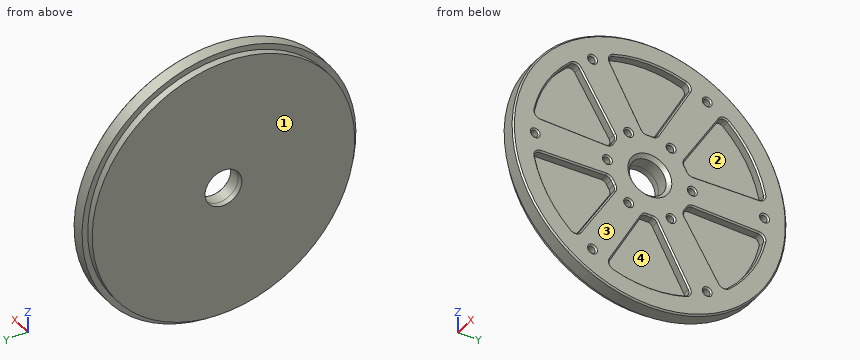
```python
from build123d import *

# Parameters (mm, degrees)
SKETCH1_R           = 48.35
BOSS_EXTRUDE1_DEPTH = 2.725
SKETCH3_R           = 1.25
CUT_EXTRUDE1_DEPTH  = 3
CIRPATTERN1_COUNT   = 6
SKETCH4_R           = 1.25
CUT_EXTRUDE2_DEPTH  = 3
CIRPATTERN2_COUNT   = 6
SKETCH5_R           = 6.5
CUT_EXTRUDE3_DEPTH  = 5.45
CHAMFER1_SIZE       = 0.5
CHAMFER2_SIZE       = 1.25
CHAMFER3_SIZE       = 0.5
SKETCH6_R           = 46.35
SKETCH6_R_2         = 6.5
BOSS_EXTRUDE2_DEPTH = 2
CUT_EXTRUDE4_START  = -0.5
SKETCH7_R           = 48.35
SKETCH7_R_2         = 46.35
CUT_EXTRUDE4_DEPTH  = 0.5
CUT_EXTRUDE6_DEPTH  = 3
CIRPATTERN3_COUNT   = 6
CHAMFER4_SIZE       = 0.5


with BuildPart() as part:
    # Sketch1 → Boss-Extrude1 (new, symmetric)
    with BuildSketch(Plane(origin=(0, 0, 0), x_dir=(0, 0, -1), z_dir=(1, 0, 0))):
        Circle(SKETCH1_R)
    extrude(amount=BOSS_EXTRUDE1_DEPTH, both=True)

    # Sketch3 → Cut-Extrude1 (cut)
    with BuildSketch(Plane(origin=(2.725, 0, 0), x_dir=(0, 0, -1), z_dir=(1, 0, 0))):
        with Locations((0, 40.5)):
            Circle(SKETCH3_R)
    cut_extrude1 = extrude(amount=-CUT_EXTRUDE1_DEPTH, mode=Mode.SUBTRACT)

    # CirPattern1: Cut-Extrude1 ×6 about axis
    cirpattern1_axis = Axis((0, 0, 0), (1, 0, 0))
    for i in range(1, CIRPATTERN1_COUNT):
        add(cut_extrude1.rotate(cirpattern1_axis, i * 360 / CIRPATTERN1_COUNT), mode=Mode.SUBTRACT)

    # Sketch4 → Cut-Extrude2 (cut)
    with BuildSketch(Plane(origin=(2.725, 0, 0), x_dir=(0, 0, -1), z_dir=(1, 0, 0))):
        with Locations((0, 15)):
            Circle(SKETCH4_R)
    cut_extrude2 = extrude(amount=-CUT_EXTRUDE2_DEPTH, mode=Mode.SUBTRACT)

    # CirPattern2: Cut-Extrude2 ×6 about axis
    cirpattern2_axis = Axis((0, 0, 0), (1, 0, 0))
    for i in range(1, CIRPATTERN2_COUNT):
        add(cut_extrude2.rotate(cirpattern2_axis, i * 360 / CIRPATTERN2_COUNT), mode=Mode.SUBTRACT)

    # Sketch5 → Cut-Extrude3 (cut)
    with BuildSketch(Plane(origin=(2.725, 0, 0), x_dir=(0, 0, -1), z_dir=(1, 0, 0))):
        Circle(SKETCH5_R)
    extrude(amount=-CUT_EXTRUDE3_DEPTH, mode=Mode.SUBTRACT)

    # Chamfer1
    chamfer1_edges = [part.edges().sort_by_distance(p)[0] for p in [
        (2.725, 19.167468245, 35.699028853),
        (2.725, -21.332531755, 34.449028853),
        (2.725, -40.5, -1.25),
        (2.725, -19.167468245, -35.699028853),
        (2.725, 21.332531755, -34.449028853),
        (2.725, 15, 1.25),
        (2.725, 8.582531755, -12.365381057),
        (2.725, -6.417468245, -13.615381057),
        (2.725, -15, -1.25),
        (2.725, -8.582531755, 12.365381057),
        (2.725, 6.417468245, 13.615381057),
        (2.725, 40.5, 1.25),
    ]]
    chamfer(chamfer1_edges, length=CHAMFER1_SIZE)

    # Chamfer2
    chamfer2_edges = [part.edges().sort_by_distance(p)[0] for p in [
        (2.725, 0, 6.5),
    ]]
    chamfer(chamfer2_edges, length=CHAMFER2_SIZE)

    # Chamfer3
    chamfer3_edges = [part.edges().sort_by_distance(p)[0] for p in [
        (2.725, 0, 48.35),
    ]]
    chamfer(chamfer3_edges, length=CHAMFER3_SIZE)

    # Sketch6 → Boss-Extrude2 (add)
    with BuildSketch(Plane.ZY.offset(2.725)):
        Circle(SKETCH6_R)
        with Locations(Location((0, 0, 0), (0, 0, 180))):
            Circle(SKETCH6_R_2, mode=Mode.SUBTRACT)
    extrude(amount=BOSS_EXTRUDE2_DEPTH)

    # Sketch7 → Cut-Extrude4 (cut)
    with BuildSketch(Plane.ZY.offset(2.725).offset(CUT_EXTRUDE4_START)):
        Circle(SKETCH7_R)
        Circle(SKETCH7_R_2, mode=Mode.SUBTRACT)
    extrude(amount=CUT_EXTRUDE4_DEPTH, mode=Mode.SUBTRACT)

    # Sketch9 → Cut-Extrude6 (cut)
    with BuildSketch(Plane(origin=(2.725, 0, 0), x_dir=(0, 0, -1), z_dir=(1, 0, 0))):
        with BuildLine():
            Line((-6.216449103, 38.533984802), (-5.619911931, 15.248157726))
            ThreePointArc((-5.619911931, 15.248157726), (-5.904066218, 14.168286857), (-6.722872915, 13.409063344))
            ThreePointArc((-6.722872915, 13.409063344), (-7.5, 12.990381057), (-8.251153039, 12.526710403))
            ThreePointArc((-8.251153039, 12.526710403), (-9.318063238, 12.197214759), (-10.395335986, 12.491065362))
            Line((-10.395335986, 12.491065362), (-30.263185196, 24.650595245))
            ThreePointArc((-30.263185196, 24.650595245), (-31.198505813, 26.069807791), (-30.704246509, 27.696060123))
            ThreePointArc((-30.704246509, 27.696060123), (-20.675, 35.810150446), (-8.633368397, 40.438687542))
            ThreePointArc((-8.633368397, 40.438687542), (-6.977862912, 40.05360249), (-6.216449103, 38.533984802))
        make_face()
    cut_extrude6 = extrude(amount=-CUT_EXTRUDE6_DEPTH, mode=Mode.SUBTRACT)

    # CirPattern3: Cut-Extrude6 ×6 about axis
    cirpattern3_axis = Axis((0, 0, 0), (1, 0, 0))
    for i in range(1, CIRPATTERN3_COUNT):
        add(cut_extrude6.rotate(cirpattern3_axis, i * 360 / CIRPATTERN3_COUNT), mode=Mode.SUBTRACT)

    # Chamfer4
    chamfer4_edges = [part.edges().sort_by_distance(p)[0] for p in [
        (2.725, 40.05360249, 6.977862912),
        (2.725, 35.810150446, 20.675),
        (2.725, 26.069807791, 31.198505813),
        (2.725, 18.570830304, 20.329260591),
        (2.725, 12.197214759, 9.318063238),
        (2.725, 12.990381057, 7.5),
        (2.725, 14.168286857, 5.904066218),
        (2.725, 26.891071264, 5.918180517),
        (2.725, -26.069807791, 31.198505813),
        (2.725, -35.810150447, 20.675),
        (2.725, -40.05360249, 6.977862912),
        (2.725, -26.891071264, 5.918180517),
        (2.725, -14.168286857, 5.904066218),
        (2.725, -12.990381057, 7.5),
        (2.725, -12.197214759, 9.318063238),
        (2.725, -18.570830304, 20.329260591),
        (2.725, 13.983794699, 38.176368726),
        (2.725, 0, 41.35),
        (2.725, -13.983794699, 38.176368726),
        (2.725, -8.32024096, 26.247441108),
        (2.725, -1.971072098, 15.222129456),
        (2.725, 0, 15),
        (2.725, 1.971072098, 15.222129456),
        (2.725, 8.32024096, 26.247441108),
        (2.725, -13.983794699, -38.176368726),
        (2.725, 0, -41.35),
        (2.725, 13.983794699, -38.176368726),
        (2.725, 8.32024096, -26.247441108),
        (2.725, 1.971072098, -15.222129456),
        (2.725, 0, -15),
        (2.725, -1.971072098, -15.222129456),
        (2.725, -8.32024096, -26.247441108),
        (2.725, -40.05360249, -6.977862912),
        (2.725, -35.810150446, -20.675),
        (2.725, -26.069807791, -31.198505813),
        (2.725, -18.570830304, -20.329260591),
        (2.725, -12.197214759, -9.318063238),
        (2.725, -12.990381057, -7.5),
        (2.725, -14.168286857, -5.904066218),
        (2.725, -26.891071264, -5.918180517),
        (2.725, 26.069807791, -31.198505813),
        (2.725, 35.810150447, -20.675),
        (2.725, 40.05360249, -6.977862912),
        (2.725, 26.891071264, -5.918180517),
        (2.725, 14.168286857, -5.904066218),
        (2.725, 12.990381057, -7.5),
        (2.725, 12.197214759, -9.318063238),
        (2.725, 18.570830304, -20.329260591),
    ]]
    chamfer(chamfer4_edges, length=CHAMFER4_SIZE)


solid = part.part
```
Geometry check sheet. Reference: the model listing, model coordinates, mm. Face numbers are marked on the shaded views. A direction names the side the tool comes from. Coordinates: 2 decimals unless noted, no trailing zeros.
Item 1: Mould release check, pull along Y, two halves, no side actions. Record for the marked faces 1 and 2: released by +Y, released by -Y, zero draft, split by the parting line, or undercut.
Item 2: Depth check by flat-ended pin: pin 1 (1.2 mm diameter, centred on y = 20.5, z = 35, fed in from +X) (3 decimals); pin 2 (2 mm diameter, centred on y = 40.5, z = 0.5, fed in from +X) (3 decimals); pin 3 (13 mm diameter, centred on y = 21, z = -18.5, fed in from +X) (3 decimals); pin 4 (4 mm diameter, centred on x = -1.5, z = -16.5, fed in from +Y). Enter the tip coordinate at first touch or a pass-through.
Item 3: Scan lines: line 1 along Y through (x, z) = (0.9, 0); line 2 along Y through (x, z) = (1.55, 0) (3 decimals); line 3 along X through (y, z) = (-25, -17) (3 decimals). Record each from-to range of solid material in increasing order.
Item 4: Tool access check on the marked faces 3 and 4. Record the directions out of +Z, -Z, +X, -X, +Y, -Y that give a thin tool (end or side, any length) a straight path to the whole face; none if there is none.
Check sheet entries:
1. face 1: zero draft
1. face 2: undercut
2. pin 1: stops at x = -0.275
2. pin 2: stops at x = 2.475
2. pin 3: stops at x = 2.725
2. pin 4: stops at y = 46.12
3. line 1: y = -48.35 to -41.75, -39.25 to -16.25, -13.75 to -6.5, 6.5 to 13.75, 16.25 to 39.25, 41.75 to 48.35
3. line 2: y = -48.35 to -41.75, -39.25 to -16.25, -13.75 to -6.575, 6.575 to 13.75, 16.25 to 39.25, 41.75 to 48.35
3. line 3: x = -4.725 to -0.275
4. face 3: +Z, -Z, +X, +Y, -Y
4. face 4: +X
